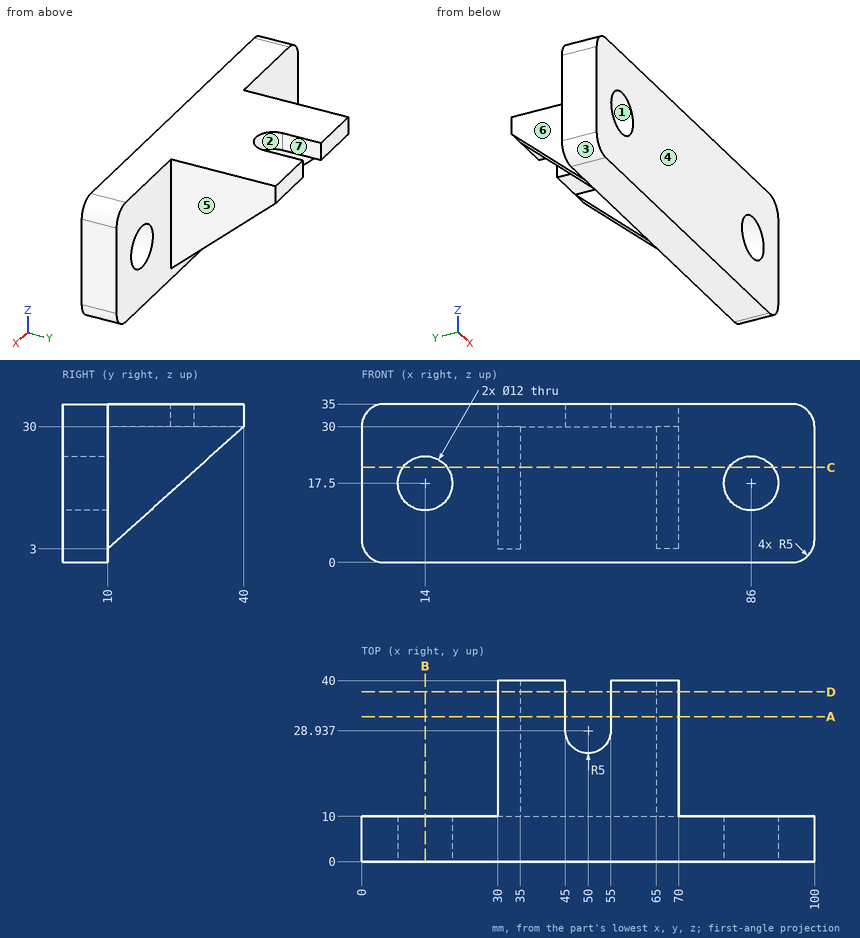
Input: dimensioned drawing with shaded views. Units: mm. Origin: part minimum x, y, z. A direction names the side the tool comes from. Coordinates: 2 decimals unless noted, no trailing zeros. Loops run counter-clockwise (first coordinate to the right, second up) from the corner with the lowest first, then second, coordinate; pieces in that order, holes last.
Q1. Section A-A, the plane y = 32. Return the cut outline in (x, z).
Results are:
outline: (30, 22.8) - (35, 22.8) - (35, 30) - (45, 30) - (45, 35) - (30, 35) - close; (55, 30) - (65, 30) - (65, 22.8) - (70, 22.8) - (70, 35) - (55, 35) - close
Q2. Section B-B, the plane x = 14. Return the cut outline in (y, z).
Results are:
outline: (0, 0) - (10, 0) - (10, 11.5) - (0, 11.5) - close; (0, 23.5) - (10, 23.5) - (10, 35) - (0, 35) - close
Q3. Mould query, pull axis X, two halves, no side actions, for the marked faces 1, 2, 3 and 4. Classes: +X half, -X half, draft (parallel to the pull), parting line (faces both ways), or undercut.
Results are:
face 1: undercut
face 2: undercut
face 3: -X half
face 4: draft
Q4. Contact query for flat-ended pins moving along their axis: pin 1 (10.5 mm diameter, centred on x = 31, z = 26, fed in from +Y); pin 2 (4 mm diameter, centred on x = 12, z = 9, fed in from +Y); pin 3 (15 mm diameter, centred on y = 32, z = 22.5, fed in from +X); pin 4 (4 mm diameter, centred on y = 29.5, z = 17, fed in from -X). Output: stop coordinate, or through.
Results are:
pin 1: stops at y = 40
pin 2: stops at y = 10
pin 3: stops at x = 70
pin 4: passes through
Q5. Section D-D, the plane y = 37.5. Return the cut outline in (x, z).
Results are:
outline: (30, 27.75) - (35, 27.75) - (35, 30) - (45, 30) - (45, 35) - (30, 35) - close; (55, 30) - (65, 30) - (65, 27.75) - (70, 27.75) - (70, 35) - (55, 35) - close
Q6. Section C-C, the plane z = 21. Return the cut outline in (x, y), and give its area (4 significant figures).
Results are:
outline: (0, 0) - (9.13, 0) - (9.13, 10) - (0, 10) - close; (18.87, 0) - (81.13, 0) - (81.13, 10) - (70, 10) - (70, 30) - (65, 30) - (65, 10) - (35, 10) - (35, 30) - (30, 30) - (30, 10) - (18.87, 10) - close; (90.87, 0) - (100, 0) - (100, 10) - (90.87, 10) - close
area: 1,005 mm2
Q7. Set-up query: the marked faces 5, 6 and 7. Return all of +Z, -Z, +X, -X, +Y, -Y with unobstructed straight access to the full face (end or side cutting, diameter ignored); none if empty.
Results are:
face 5: +Z, -Z, +X, +Y
face 6: +Z, -Z, -X, +Y
face 7: +Z, -Z, +Y
Q8. Line query: line 1 along X through (y, z) = (5, 17); line 2 along X through (y, z) = (37, 28); line 3 along X through (y, z) = (5, 15) (1 decimal). Output: solid intervals per line, ascending.
Results are:
line 1: x = 0 to 8.02, 19.98 to 80.02, 91.98 to 100
line 2: x = 30 to 35, 65 to 70
line 3: x = 0 to 8.5, 19.5 to 80.5, 91.5 to 100
